Model file for the job. Use its own axes, mm. Face numbers are marked on the shaded views. A direction names the side the tool comes from. Round coordinates to 2 decimals unless told otherwise and drop trailing zeros. Order: outer loops, then holes, each group sorted by start corner. A loop starts at its lowest first (then second) coordinate and runs counter-clockwise, first axis right, second up. Notation, with made-up numbers: (23, 23) -> (34, 23) arc R12 cw to (34, 31) -> close; hole circle Ø8 at (20, 71.25). An arc over 180 degrees is marked (long way). Answer as CSV lines item,"result".
Autodesk Inventor part; units mm, degrees
ref_plane "YZ Plane" through (0, 0, 0) normal (1, 0, 0) x (0, 1, 0)
ref_plane "XZ Plane" through (0, 0, 0) normal (0, 1, 0) x (-1, 0, 0)
ref_plane "XY Plane" through (0, 0, 0) normal (0, 0, 1) x (1, 0, 0)
sketch "Sketch1" plane through (0, 0, 0) normal (0, 1, 0) x (-1, 0, 0)
  line L0 (8.5, 21.5) -> (-8.5, 21.5) construction
  line L1 (-8.5, 21.5) -> (-8.5, -21.5) construction
  line L2 (8.5, -21.5) -> (8.5, 21.5) construction
  line L3 (-8.5, 21.5) -> (8.5, -21.5) construction
  line L4 (-8.5, -21.5) -> (8.5, 21.5) construction
  line L5 (-3.5, -21.5) -> (-3.5, -23.5) construction
  line L6 (-3.5, -23.5) -> (3.5, -23.5) construction
  line L7 (3.5, -23.5) -> (3.5, -21.5) construction
  line L8 (-8.5, -21.5) -> (-3.5, -21.5) construction
  line L9 (3.5, -21.5) -> (8.5, -21.5) construction
  arc A0 (9.5253, -23.1034) -> (-9.5253, -23.1034) centre (0, 0) ccw
  line L10 (9.5253, -23.1034) -> (-9.5253, -23.1034)
  line L11 (-10.102, -26.1034) -> (10.102, -26.1034)
  arc A1 (10.102, -26.1034) -> (-10.102, -26.1034) centre (0, 0) ccw
  dimension "d0" = 43
  dimension "d1" = 17
  dimension "d2" = 7
  dimension "d3" = 2
  dimension "d4" = 3
  dimension "d13" = 20.204
extrude "BASE PLATE" add sketch "Sketch1" along normal blind 3 contours L10 A0 | A1 L11
sketch "Sketch3" plane through (0, 3, 0) normal (0, 1, 0) x (1, 0, 0)
  line L0 (10.102, 26.1034) -> (-10.102, 26.1034)
  arc A0 (-10.102, 26.1034) -> (10.102, 26.1034) centre (0, 0) ccw
  arc A1 (-10.102, 26.1034) -> (10.102, 26.1034) centre (0, 0) ccw
  line L1 (-10.102, 26.1034) -> (10.102, 26.1034)
  circle A2 centre (0, 0) radius 24.99
  dimension "d58" = 3
extrude "WALLS" add sketch "Sketch3" along normal blind 10
sketch "Sketch6" plane through (0, 3, 0) normal (0, 1, 0) x (1, 0, 0)
  line L0 (-8.5, 21.5) -> (8.5, 21.5) construction
  line L1 (8.5, 21.5) -> (8.5, -21.5) construction
  line L2 (8.5, -21.5) -> (-8.5, -21.5) construction
  line L3 (-8.5, -21.5) -> (-8.5, 21.5) construction
  line L4 (-8.5, -21.5) -> (8.5, 21.5) construction
  line L5 (-8.5, 21.5) -> (8.5, -21.5) construction
  line L6 (0, 0) -> (-15, 0) construction
  line L7 (-15, 0) -> (-15, 10) construction
  line L8 (-15, 10) -> (0, 10) construction
  line L9 (0, 10) -> (0, 0) construction
  circle A0 centre (-15, 10) radius 4
  circle A1 centre (-15, 10) radius 2.5
  circle A2 centre (-15, -10) radius 4
  circle A3 centre (-15, -10) radius 2.5
  circle A4 centre (15, 10) radius 4
  circle A5 centre (15, 10) radius 2.5
  circle A6 centre (15, -10) radius 2.5
  circle A7 centre (15, -10) radius 4
  dimension "d18" = 43
  dimension "d19" = 17
  dimension "d20" = 15
  dimension "d21" = 10
  dimension "d22" = 8
  dimension "d23" = 5
extrude "BUTTON POSTS" add sketch "Sketch6" along normal blind 7
sketch "Sketch7" plane through (0, 3, 0) normal (0, 1, 0) x (1, 0, 0)
  line L0 (-9, 24.1034) -> (9, 24.1034)
  line L1 (9, 24.1034) -> (9, -19.0966)
  line L2 (9, -19.0966) -> (-9, -19.0966)
  line L3 (-9, -19.0966) -> (-9, 24.1034)
  line L4 (-17, 3.75) -> (-13, 3.75)
  line L5 (-13, 3.75) -> (-13, -3.75)
  line L6 (-13, -3.75) -> (-17, -3.75)
  line L7 (-17, -3.75) -> (-17, 3.75)
  line L8 (-24.99, 0) -> (24.99, 0) construction
  line L9 (0, 23.1034) -> (0, -24.99) construction
  line L10 (17, 3.75) -> (13, 3.75)
  line L11 (13, 3.75) -> (13, -3.75)
  line L12 (13, -3.75) -> (17, -3.75)
  line L13 (17, -3.75) -> (17, 3.75)
  line L14 (-9.5253, 24.1034) -> (9.5253, 24.1034)
  line L15 (10.102, 26.1034) -> (-10.102, 26.1034)
  dimension "d26" = 43.2
  dimension "d27" = 18
  dimension "d28" = 7.5
  dimension "d29" = 4
  dimension "d30" = 3.75
  dimension "d63" = 2
  dimension "d65" = 9
  dimension "d77" = 13
extrude "INDENTATION FOR LINEUP" cut sketch "Sketch7" against normal blind 1
sketch "Sketch9" plane through (0, 2, 0) normal (0, 1, 0) x (1, 0, 0)
  line L0 (-9, 24.1034) -> (9, 24.1034)
  line L1 (-9, -19.0966) -> (9, -19.0966)
  line L2 (9, -19.0966) -> (9, 24.1034)
  line L3 (9, 24.1034) -> (-9, 24.1034)
  line L4 (-9, 24.1034) -> (-9, -19.0966)
  point P0 (0, 0)
extrude "FLAT SURFACE FOR ARDUINO" cut sketch "Sketch9" along normal blind 8
sketch "Sketch11" plane through (10.102, 0, -26.1034) normal (0, 0, -1) x (-1, 0, 0)
  line L0 (19.102, 2) -> (1.102, 2) construction
  line L1 (0, 0) -> (0, 13) construction
  line L2 (20.204, 0) -> (20.204, 13) construction
  line L3 (6.1, 10) -> (14.1, 10)
  line L4 (14.1, 10) -> (14.1, 6)
  line L5 (14.1, 6) -> (6.1, 6)
  line L6 (6.1, 6) -> (6.1, 10)
  line L7 (0, 0) -> (20.204, 0) construction
  circle A0 centre (2.5, 9.5) radius 1
  point P0 (10.102, 0)
  dimension "d69" = 4
  dimension "d70" = 4
  dimension "d71" = 6.1
  dimension "d72" = 2
  dimension "d74" = 2.5
  dimension "d78" = 7.5
  dimension "d89" = 8
extrude "I/O HOLES" cut sketch "Sketch11" against normal blind 10
sketch "Sketch12" plane through (0, 3, 0) normal (0, 1, 0) x (1, 0, 0)
  line L0 (19.1097, 16.1034) -> (9, 16.1034)
  line L1 (9, 16.1034) -> (9, 23.3131)
  line L2 (-9, 24.1034) -> (9, 24.1034) construction
  line L3 (-9, -19.0966) -> (-9, 24.1034) construction
  line L4 (9, -19.0966) -> (-9, -19.0966) construction
  line L5 (9, 24.1034) -> (9, -19.0966) construction
  line L6 (10.102, 26.1034) -> (-10.102, 26.1034)
  circle A0 centre (0, 0) radius 24.99 construction
  arc A1 (-9, 23.3131) -> (9, 23.3131) centre (0, 0) ccw
  arc A2 (19.1097, 16.1034) -> (9, 23.3131) centre (0, 0) ccw
  line L7 (9, 23.3131) -> (9, -19.0966)
  point P0 (13, 21.3424)
  dimension "d88" = 10
extrude "Extrusion11" add sketch "Sketch12" along normal blind 7
sketch "Sketch15" plane through (0, 10, 0) normal (0, 1, 0) x (1, 0, 0)
  line L0 (9, 23.3131) -> (9, 16.1034) construction
  line L1 (9, 16.1034) -> (19.1097, 16.1034) construction
  arc A0 (19.1097, 16.1034) -> (9, 23.3131) centre (0, 0) ccw construction
  line L2 (6.602, 26.1034) -> (8.602, 26.1034) construction
  line L3 (8.468, 24.1034) -> (6.736, 24.1034) construction
  line L4 (7.602, 26.1034) -> (7.602, 18.0057) construction
  line L5 (5.602, 19.8034) -> (9.602, 19.8034) construction
  line L6 (9.602, 19.8034) -> (9.602, 18.1034) construction
  line L7 (9.602, 18.1034) -> (5.602, 18.1034) construction
  line L8 (5.602, 18.1034) -> (5.602, 19.8034) construction
  line L9 (9, 19.8034) -> (9.602, 19.8034)
  line L10 (9.602, 19.8034) -> (9.602, 18.1034)
  line L11 (9.602, 18.1034) -> (9, 18.1034)
  line L12 (9, 18.1034) -> (9, 19.8034)
  line L13 (8.468, 23.5115) -> (8.468, 24.1034)
  line L14 (6.736, 24.1034) -> (6.736, 24.065)
  point P0 (8.602, 24.1034)
  point P1 (6.602, 24.1034)
  point P2 (9, 19.7083)
  dimension "d90" = 4
  dimension "d91" = 2
  dimension "d92" = 1.7
  dimension "d93" = 2
extrude "Extrusion12" cut sketch "Sketch15" against normal blind 2.3
sketch "Sketch16" plane through (9, 2, -24.1034) normal (-1, 0, 0) x (0, 0, 1)
  line L0 (0, 8) -> (0, 6.5) construction
  line L1 (6, 8) -> (8, 8) construction
  line L2 (6, 8) -> (6, 5.7) construction
  line L3 (6, 5.7) -> (4.3, 5.7) construction
  line L4 (4.3, 5.7) -> (4.3, 8) construction
  line L5 (0.7903, 8) -> (4.3, 8) construction
  line L6 (8, 1) -> (8, 8) construction
  line L7 (6, 8) -> (8, 8) construction
  line L8 (14.8538, 7.25) -> (0, 7.25) construction
  line L9 (0, 0) -> (0, 8) construction
  line L10 (6, 8) -> (8, 8)
  line L11 (8, 8) -> (8, 5)
  line L12 (8, 5) -> (6, 5)
  line L13 (6, 5) -> (6, 8)
  point P0 (24.1034, -2)
  dimension "d96" = 3
  dimension "d97" = 2
extrude "Extrusion13" add sketch "Sketch16" along normal blind 4.398
sketch "Sketch17" plane through (9.602, 7.7, -18.1034) normal (0, 0, -1) x (-1, 0, 0)
  line L0 (5, -0.7) -> (4.2, -0.7)
  line L1 (4.2, -0.7) -> (4.2, 2.3)
  line L2 (4.2, 2.3) -> (5, 2.3)
  line L3 (5, 2.3) -> (5, -0.7)
  point P0 (9.602, -7.7)
  dimension "d100" = 3
  dimension "d101" = 0.8
extrude "Extrusion14" add sketch "Sketch17" along normal blind 2
equation "\"d30\" = 0.5 * d28"
equation "\"d65\" = 0.5 * d27"
equation "\"d91\" = 0.5 * d90"
properties part number "Base"
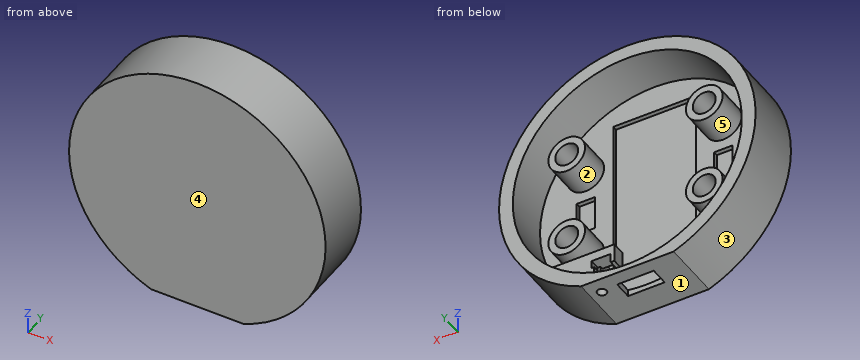
Q1. Flat gauge pins, fed straight in: pin 1 (1.5 mm diameter, centred on x = 16, z = -9.5, fed in from +Y); pin 2 (4 mm diameter, centred on y = 6, z = -12, fed in from +X); pin 3 (1.1 mm diameter, centred on y = 2.5, z = 2, fed in from +X). Where does each tip first touch, or does it go through?
Checks:
pin 1,"y = 3"
pin 2,"x = 26.14"
pin 3,"x = 27.95"
Q2. Saw through at C-C (x = 3). Write the cut outline in (y, z), plus the area to 3 significant figures.
Checks:
outline,"(0, -26.1) -> (6, -26.1) -> (6, -24.81) -> (3, -24.81) -> (3, -24.1) -> (2, -24.1) -> (2, 19.1) -> (3, 19.1) -> (3, 24.81) -> (13, 24.81) -> (13, 27.83) -> (0, 27.83) -> close; (10, -26.1) -> (13, -26.1) -> (13, -24.81) -> (10, -24.81) -> close"
area,"157 mm²"
Q3. Saw through at D-D (x = -15). Write the cut outline in (y, z), plus the area to 3 significant figures.
Checks:
outline,"(0, -23.63) -> (13, -23.63) -> (13, -19.99) -> (3, -19.99) -> (3, -14) -> (10, -14) -> (10, -12.5) -> (3, -12.5) -> (3, -7.5) -> (10, -7.5) -> (10, -6) -> (3, -6) -> (3, -3.75) -> (2, -3.75) -> (2, 3.75) -> (3, 3.75) -> (3, 6) -> (10, 6) -> (10, 7.5) -> (3, 7.5) -> (3, 12.5) -> (10, 12.5) -> (10, 14) -> (3, 14) -> (3, 19.99) -> (13, 19.99) -> (13, 23.63) -> (0, 23.63) -> close"
area,"249 mm²"
Q4. Tool access for the marked faces 1 and 2: list every direction of +Z, -Z, +X, -X, +Y, -Y with a clear straight run to the whole face (end or side of a thin tool).
Checks:
face 1,"-Z, +X, -X, +Y, -Y"
face 2,"+Y"
Q5. Wall check: L1, parallel to X at y = 7, z = -10; L2, parallel to Z at x = -15, y = 8.5; L3, parallel to X at y = 6.75, z = -12. Give the ranges that are in metal, low to high. Write a range as [from, to].
Checks:
L1,"[-26.14, -22.9], [-19, -17.5], [-12.5, -11], [11, 12.5], [17.5, 19], [22.9, 26.14]"
L2,"[-23.63, -19.99], [-14, -12.5], [-7.5, -6], [6, 7.5], [12.5, 14], [19.99, 23.63]"
L3,"[-25.29, -21.92], [-18.46, -16.5], [-13.5, -11.54], [11.54, 13.5], [16.5, 18.46], [21.92, 25.29]"
Q6. Saw through at A-A (y = 4.75). State how many separate pieces and enclosed holes the cut face has, plus the area to 3 significant figures.
Checks:
separate pieces,"5"
enclosed holes,"5"
area,"637 mm²"
Q7. Mould opens along Z. For the marked faces 3, 4 and 5 say: +Z half, -Z half, draft (parallel to the pull), parting line (faces both ways), or undercut.
Checks:
face 3,"parting line"
face 4,"draft"
face 5,"undercut"
Q8. Saw through at B-B (z = 0). Write the cut outline in (x, y), plus the area to 3 significant figures.
Checks:
outline,"(-27.99, 0) -> (27.99, 0) -> (27.99, 13) -> (24.99, 13) -> (24.99, 3) -> (17, 3) -> (17, 2) -> (13, 2) -> (13, 3) -> (9, 3) -> (9, 2) -> (-9, 2) -> (-9, 3) -> (-13, 3) -> (-13, 2) -> (-17, 2) -> (-17, 3) -> (-24.99, 3) -> (-24.99, 13) -> (-27.99, 13) -> close"
area,"202 mm²"
